from build123d import *

# Parameters (mm, degrees)
F0_W      = 165
F0_H      = 45
F0_R      = 12.5
F1_DEPTH  = 1
F3_DEPTH  = 1
F4_DEPTH  = 25
F5_DEPTH  = 25
F6_R      = 13.5
F6_R_2    = 12.5
F7_DEPTH  = 5
F8_R      = 13.5
F8_R_2    = 5
F9_DEPTH  = 1
F11_DEPTH = 1


with BuildPart() as f1:
    # F0 (on Front) → F1 (new body)
    with BuildSketch(Plane.XZ):
        Rectangle(F0_W, F0_H)
        with Locations((-65, 0)):
            Circle(F0_R, mode=Mode.SUBTRACT)
        with Locations((65, 0)):
            Circle(F0_R, mode=Mode.SUBTRACT)
    extrude(amount=F1_DEPTH)

    # F2 (on face) → F3 (join)
    with BuildSketch(Plane.XZ.offset(1)):
        with BuildLine():
            Line((68.3925151825, -19.0988145769), (65, -22.5))
            ThreePointArc((65, -22.5), (87.5, 0), (65, 22.5))
            Line((65, 22.5), (71.474224329, 16.2770561874))
            Line((71.474224329, 16.2770561874), (77.4062722921, 9.1145541519))
            Line((77.4062722921, 9.1145541519), (80.3926512599, 2.1407562308))
            Line((80.3926512599, 2.1407562308), (80.3926512599, -5.2317115478))
            Line((80.3926512599, -5.2317115478), (78.3914923668, -12.1520543471))
            Line((78.3914923668, -12.1520543471), (74.6632069349, -14.4081749022))
            Line((74.6632069349, -14.4081749022), (68.3925151825, -19.0988145769))
        make_face()
        with BuildLine():
            Line((-65, 14.9617949501), (-65, 22.5))
            ThreePointArc((-65, 22.5), (-87.5, 0), (-65, -22.5))
            Line((-65, -22.5), (-67.4760043621, -15.6979020685))
            Line((-67.4760043621, -15.6979020685), (-72.8440880775, -12.9142012447))
            Line((-72.8440880775, -12.9142012447), (-76.5851810575, -7.8018400818))
            Line((-76.5851810575, -7.8018400818), (-79.5639529824, 0))
            Line((-79.5639529824, 0), (-79.5639529824, 6.4657721668))
            Line((-79.5639529824, 6.4657721668), (-75.4495188594, 11.7608513683))
            Line((-75.4495188594, 11.7608513683), (-65, 14.9617949501))
        make_face()
    extrude(amount=-F3_DEPTH)

    # F2 (on face) → F4 (cut)
    with BuildSketch(Plane.XZ.offset(1)):
        with BuildLine():
            Line((-82.5, 22.5), (-82.5, 14.1421356237))
            ThreePointArc((-82.5, 14.1421356237), (-74.6966991411, 20.3033008589), (-65, 22.5))
            Line((-65, 22.5), (-82.5, 22.5))
        make_face()
    extrude(amount=-F4_DEPTH, mode=Mode.SUBTRACT)

    # F2 (on face) → F5 (cut)
    with BuildSketch(Plane.XZ.offset(1)):
        with BuildLine():
            ThreePointArc((82.5, -14.1421356237), (74.6966991411, -20.3033008589), (65, -22.5))
            Line((65, -22.5), (82.5, -22.5))
            Line((82.5, -22.5), (82.5, -14.1421356237))
        make_face()
        with BuildLine():
            ThreePointArc((65, 22.5), (74.6966991411, 20.3033008589), (82.5, 14.1421356237))
            Line((82.5, 14.1421356237), (82.5, 22.5))
            Line((82.5, 22.5), (65, 22.5))
        make_face()
        with BuildLine():
            Line((-82.5, -22.5), (-65, -22.5))
            ThreePointArc((-65, -22.5), (-74.6966991411, -20.3033008589), (-82.5, -14.1421356237))
            Line((-82.5, -14.1421356237), (-82.5, -22.5))
        make_face()
    extrude(amount=-F5_DEPTH, mode=Mode.SUBTRACT)

    # F6 (on face) → F7 (join)
    with BuildSketch(Plane.XZ.offset(1)):
        with Locations((-65, 0)):
            Circle(F6_R)
        with Locations((-65, 0)):
            Circle(F6_R_2, mode=Mode.SUBTRACT)
        with Locations((65, 0)):
            Circle(F6_R)
        with Locations((65, 0)):
            Circle(F6_R_2, mode=Mode.SUBTRACT)
    extrude(amount=F7_DEPTH)

    # F8 (on face) → F9 (join)
    with BuildSketch(Plane.XZ.offset(6)):
        with Locations((-65, 0)):
            Circle(F8_R)
        with Locations((-65, 0)):
            Circle(F8_R_2, mode=Mode.SUBTRACT)
        with Locations((65, 0)):
            Circle(F8_R)
        with Locations((65, 0)):
            Circle(F8_R_2, mode=Mode.SUBTRACT)
    extrude(amount=F9_DEPTH)

    # F10 (on face) → F11 (join)
    with BuildSketch(Plane.XZ.offset(1)):
        Polygon((-81.9395110011, 0), (-87.5, 0), (-87.5, -22.5), (-65, -22.5), (-65, -18.5897927731), (-73.3228996396, -16.0001199692), (-80.1934376359, -9.6208481118), align=None)
    extrude(amount=-F11_DEPTH)


solid = f1.part
The model under review builds one solid part; all positions refer to its coordinate system, in mm. A direction names the side the tool comes from. Round coordinates to 2 decimals unless told otherwise and drop trailing zeros. Order: outer loops, then holes, each group sorted by start corner. A loop starts at its lowest first (then second) coordinate and runs counter-clockwise, first axis right, second up. Notation, with made-up numbers: (88, 72) -> (137, 72) arc R28 cw to (137, 96) -> close; hole circle Ø2 at (-15, -30). An arc over 180 degrees is marked (long way). Return JSON: item names as keys, results as strings.
1. For L1, parallel to Z at x = 65, y = -6.3; L2, parallel to X at y = -3.25, z = 5; L3, parallel to Z at x = -65, y = -3.3, list the stretches that pass through material, from the lowest coordinate up. Write a range as [from, to].
Answer block:
{"L1": "z = [-13.5, -5], [5, 13.5]", "L2": "x = [-77.54, -76.46], [-53.54, -52.46], [52.46, 53.54], [76.46, 77.54]", "L3": "z = [-13.5, -12.5], [12.5, 13.5]"}
2. The part is to be moulded in two halves that separate along Z. For faces 1 (the face through (51.513, -3.958, 0.594)), 2 (the face through (64.8, -6, -5.4)), 3 (the face through (-1, -1, 0)), say which applies: +Z half, -Z half, draft (parallel to the pull), parting line (faces both ways), or undercut.
Answer block:
{"face 1": "parting line", "face 2": "undercut", "face 3": "draft"}
3. For faces 4 (the face through (-78.487, -3.958, 0.594)), 5 (the face through (-77.488, -2.958, 0.55)), 6 (the face through (71, -7, 0)), list the 3-axis set-ups (+Z, -Z, +X, -X, +Y, -Y) from which the entire face can be reached by the end or side of a thin tool; tool diameter is ignored.
Answer block:
{"face 4": "-Y", "face 5": "+Y", "face 6": "+Z, -Z, +X, -X, -Y"}
4. Take a section at B-B (x = 17.5). Write out the cut boundary in (y, z).
Answer block:
{"outline": "(-1, -22.5) -> (0, -22.5) -> (0, 22.5) -> (-1, 22.5) -> close"}
5. Insertion check: P1, Ø4, axis at x = -66.5, y = -2.5, coming from the +Z side; P2, Ø1.5, axis at x = -11, y = -2, coming from the +Z side; P3, Ø13.5, axis at x = 22, z = -0.5, coming from the -Y side; P4, Ø1.5, axis at y = -3.5, z = 1.5, coming from the -X side. Each pin has a flat end and moves straight along its axis. Give the tip position at first contact, or say it passes through.
Answer block:
{"P1": "stops at z = 22.5", "P2": "passes through", "P3": "stops at y = -1", "P4": "stops at x = -78.48"}
6. Take a section at A-A (z = -3.5). Write out the cut boundary in (x, y).
Answer block:
{"outline": "(-87.5, -1) -> (-78.04, -1) -> (-78.04, -7) -> (-68.57, -7) -> (-68.57, -6) -> (-77, -6) -> (-77, 0) -> (-87.5, 0) -> close; (-61.43, -7) -> (-51.96, -7) -> (-51.96, -1) -> (51.96, -1) -> (51.96, -7) -> (61.43, -7) -> (61.43, -6) -> (53, -6) -> (53, 0) -> (-53, 0) -> (-53, -6) -> (-61.43, -6) -> close; (68.57, -7) -> (78.04, -7) -> (78.04, -1) -> (87.23, -1) -> (87.23, 0) -> (77, 0) -> (77, -6) -> (68.57, -6) -> close"}
7. Take a section at D-D (z = -11). Write out the cut boundary in (x, y).
Answer block:
{"outline": "(-87.5, -1) -> (-72.83, -1) -> (-72.83, -7) -> (-57.17, -7) -> (-57.17, -1) -> (57.17, -1) -> (57.17, -7) -> (72.83, -7) -> (72.83, -1) -> (84.63, -1) -> (84.63, 0) -> (70.94, 0) -> (70.94, -6) -> (59.06, -6) -> (59.06, 0) -> (-59.06, 0) -> (-59.06, -6) -> (-70.94, -6) -> (-70.94, 0) -> (-87.5, 0) -> close"}
8. Take a section at C-C (z = 18). Write out the cut boundary in (x, y), then the cut area to 3 significant figures.
Answer block:
{"outline": "(-78.5, -1) -> (78.5, -1) -> (78.5, 0) -> (-78.5, 0) -> close", "area": "157 mm²"}
